```python
from build123d import *

# Parameters (mm, degrees)
SKETCH1_R           = 1.7859375
BOSS_EXTRUDE1_DEPTH = 1.5875
FILLET1_R           = 3.571875


with BuildPart() as part:
    # Sketch1 → Boss-Extrude1 (new body)
    with BuildSketch(Plane.XY):
        with BuildLine():
            ThreePointArc((41.275, -12.7), (44.846875, -9.128125), (41.275, -5.55625))
            ThreePointArc((41.275, -5.55625), (46.83125, 0), (41.275, 5.55625))
            Line((41.275, 5.55625), (35.489019559, 5.55625))
            ThreePointArc((35.489019559, 5.55625), (32.804229109, 11.484009389), (30.119438658, 5.55625))
            Line((30.119438658, 5.55625), (11.155561342, 5.55625))
            ThreePointArc((11.155561342, 5.55625), (8.470770891, 11.484009389), (5.785980441, 5.55625))
            Line((5.785980441, 5.55625), (0, 5.55625))
            ThreePointArc((0, 5.55625), (-5.55625, 0), (0, -5.55625))
            ThreePointArc((0, -5.55625), (-3.571875, -9.128125), (0, -12.7))
            ThreePointArc((0, -12.7), (8.980256121, -8.980256121), (12.7, 0))
            Line((12.7, 0), (28.575, 0))
            ThreePointArc((28.575, 0), (32.294743879, -8.980256121), (41.275, -12.7))
        make_face()
        with BuildLine():
            ThreePointArc((0, -10.9140625), (-1.7859375, -9.128125), (0, -7.3421875))
            ThreePointArc((0, -7.3421875), (5.413228446, -4.960309977), (7.31424826, 0.639913805))
            ThreePointArc((7.31424826, 0.639913805), (8.937735019, 2.574709983), (10.872531197, 0.951223224))
            ThreePointArc((10.872531197, 0.951223224), (8.046690934, -7.37343375), (0, -10.9140625))
        make_face(mode=Mode.SUBTRACT)
        with BuildLine():
            ThreePointArc((33.96075174, 0.639913805), (35.861771554, -4.960309977), (41.275, -7.3421875))
            ThreePointArc((41.275, -7.3421875), (43.0609375, -9.128125), (41.275, -10.9140625))
            ThreePointArc((41.275, -10.9140625), (33.228309066, -7.37343375), (30.402468803, 0.951223224))
            ThreePointArc((30.402468803, 0.951223224), (32.337264981, 2.574709983), (33.96075174, 0.639913805))
        make_face(mode=Mode.SUBTRACT)
        Circle(SKETCH1_R, mode=Mode.SUBTRACT)
        with Locations((8.470770891, 7.912134389)):
            Circle(SKETCH1_R, mode=Mode.SUBTRACT)
        with Locations((41.275, 0)):
            Circle(SKETCH1_R, mode=Mode.SUBTRACT)
        with Locations((32.804229109, 7.912134389)):
            Circle(SKETCH1_R, mode=Mode.SUBTRACT)
    extrude(amount=BOSS_EXTRUDE1_DEPTH)

    # Fillet1
    fillet1_edges = [part.edges().sort_by_distance(p)[0] for p in [
        (5.785980441, 5.55625, 0.79375),
        (11.155561342, 5.55625, 0.79375),
        (30.119438658, 5.55625, 0.79375),
        (35.489019559, 5.55625, 0.79375),
        (41.275, -5.55625, 0.79375),
        (28.575, 0, 0.79375),
        (12.7, 0, 0.79375),
        (0, -5.55625, 0.79375),
    ]]
    fillet(fillet1_edges, radius=FILLET1_R)


solid = part.part
```
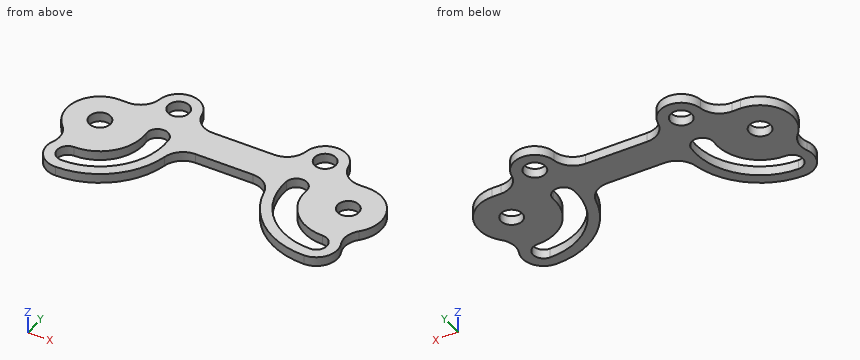
Here's how the part is built. I have some questions about the finished solid (model axes, mm). Give positions to 0.01 mm unless a question says otherwise; leave off trailing zeros. Write each loop counter-clockwise with the first axis right and the second up, starting at its lowest first coordinate (ties: lowest second). Pieces come first, ordered by that corner, then holes. Notation, with made-up numbers: M 4.5,26.25 L 22.5,26.25 A18 cw 22.5,60.25 Z; hole C -17.5,61 d11. An arc over 180 degrees is marked long. Put each result on its own line as item: value. Start each with the question number.
Item 1: I need wall thicknesses on L1, parallel to X at y = 7.25, z = 1.3; L2, parallel to Y at x = -1.5, z = 0.9; L3, parallel to Y at x = 40, z = 0.25. Which ranges of each line are inside material? Lowest first, please. Write a range as from..to.
Item 2: If we section it at C-C, the plane y = -1: Write out the boundary of the cut face in (x, z), then the cut area to 3 significant figures.
Item 3: Will these pins go through, and if not, where does the flat tip stop? pin 1 (3 mm diameter, centred on x = 0, y = 0, fed in from +Z); pin 2 (0.7 mm diameter, centred on x = 41, z = 1, fed in from +Y).
Item 4: If we section it at B-B, the plane x = 3.5: Write out the boundary of the cut face in (y, z), then the cut area to 3 significant figures.
Item 5: If we section it at D-D, the plane x = 18: Write out the boundary of the cut face in (y, z).
Item 6: If we section it at A-A, the plane y = -8.75: Write out the boundary of the cut face in (x, z), then the cut area to 3 significant figures.
Values:
1. L1: 4.47..6.81, 10.13..12.47, 28.8..31.15, 34.46..36.81
1. L2: -12.37..-10.1, -8.16..-0.97, 0.97..5.35
1. L3: -12.64..-10.84, -7.23..-1.25, 1.25..5.56
2. outline: M -5.47,0 L -1.48,0 L -1.48,1.59 L -5.47,1.59 Z; M 1.48,0 L 7.27,0 L 7.27,1.59 L 1.48,1.59 Z; M 10.87,0 L 13.4,0 L 13.4,1.59 L 10.87,1.59 Z; M 27.88,0 L 30.41,0 L 30.41,1.59 L 27.88,1.59 Z; M 34,0 L 39.8,0 L 39.8,1.59 L 34,1.59 Z; M 42.75,0 L 46.74,0 L 46.74,1.59 L 42.75,1.59 Z
2. area: 39.1 mm²
3. pin 1: through
3. pin 2: y = 5.56
4. outline: M -12.21,0 L -10.34,0 L -10.34,1.59 L -12.21,1.59 Z; M -6.45,0 L 6.22,0 L 6.22,1.59 L -6.45,1.59 Z
4. area: 23.1 mm²
5. outline: M 0,0 L 5.56,0 L 5.56,1.59 L 0,1.59 Z
6. outline: M -3.55,0 L -1.75,0 L -1.75,1.59 L -3.55,1.59 Z; M 6.52,0 L 9.2,0 L 9.2,1.59 L 6.52,1.59 Z; M 32.07,0 L 34.75,0 L 34.75,1.59 L 32.07,1.59 Z; M 43.02,0 L 44.83,0 L 44.83,1.59 L 43.02,1.59 Z
6. area: 14.2 mm²
